Can you work these out from the model? Positions are in its coordinate system, mm. A direction names the side the tool comes from. Give positions to 0.01 mm unless a question says otherwise; leave off trailing zeros. Loops run counter-clockwise (first coordinate to the right, second up) from the corner with the lowest first, then second, coordinate; pieces in that order, holes last. Notation, with made-up numbers: (18.5, -25) - (51.5, -25) arc R34 ccw to (51.5, 14) - close; hole circle Ø11 at (34.25, 75.25). An arc over 180 degrees is marked (long way). Answer in a Markdown table with one row per item.
from build123d import *

# Parameters (mm, degrees)
BOSS_EXTRUDE1_DEPTH = 3.3
BOSS_EXTRUDE2_DEPTH = 2
SKETCH5_W           = 10
SKETCH5_H           = 1.55
BOSS_EXTRUDE3_DEPTH = 0.45
SKETCH6_W           = 10
SKETCH6_H           = 1.55
BOSS_EXTRUDE4_DEPTH = 0.45
SKETCH7_W           = 10
SKETCH7_H           = 1.55
BOSS_EXTRUDE5_DEPTH = 0.45
SKETCH8_W           = 10
SKETCH8_H           = 1.55
BOSS_EXTRUDE6_DEPTH = 0.45
SKETCH9_W           = 30
SKETCH9_H           = 1.55
BOSS_EXTRUDE7_DEPTH = 0.45
SKETCH10_W          = 10
SKETCH10_H          = 1.55
BOSS_EXTRUDE8_DEPTH = 0.45
CHAMFER1_SIZE       = 0.2
SKETCH11_W          = 37.2
SKETCH11_H          = 23
CUT_EXTRUDE1_DEPTH  = 1.6
FILLET1_R           = 0.2


with BuildPart() as part:
    # Sketch1 → Boss-Extrude1 (new body)
    with BuildSketch(Plane(origin=(0, 0, 0), x_dir=(1, 0, 0), z_dir=(0, 1, 0))):
        with BuildLine():
            Line((19.586290833, 59.977163541), (19.586290833, 47.727163541))
            ThreePointArc((19.586290833, 47.727163541), (18.956570412, 46.206883961), (17.436290833, 45.577163541))
            Line((17.436290833, 45.577163541), (-0.413709167, 45.577163541))
            Line((-0.413709167, 45.577163541), (-0.413709167, 5.877163541))
            Line((-0.413709167, 5.877163541), (80.286290833, 5.877163541))
            Line((80.286290833, 5.877163541), (80.286290833, 45.577163541))
            Line((80.286290833, 45.577163541), (62.436290833, 45.577163541))
            ThreePointArc((62.436290833, 45.577163541), (60.916011253, 46.206883961), (60.286290833, 47.727163541))
            Line((60.286290833, 47.727163541), (60.286290833, 59.977163541))
            ThreePointArc((60.286290833, 59.977163541), (59.744438378, 61.285311086), (58.436290833, 61.827163541))
            Line((58.436290833, 61.827163541), (21.436290833, 61.827163541))
            ThreePointArc((21.436290833, 61.827163541), (20.128143288, 61.285311086), (19.586290833, 59.977163541))
        make_face()
    extrude(amount=BOSS_EXTRUDE1_DEPTH)

    # Sketch2 → Boss-Extrude2 (add)
    with BuildSketch(Plane(origin=(0, 3.3, 0), x_dir=(1, 0, 0), z_dir=(0, 1, 0))):
        with BuildLine():
            Line((57.136290833, -1.272836459), (65.436290833, -1.272836459))
            Line((65.436290833, -1.272836459), (80.761323353, 1.251286544))
            ThreePointArc((80.761323353, 1.251286544), (81.961096565, 1.930492929), (82.436290833, 3.224698275))
            Line((82.436290833, 3.224698275), (82.436290833, 45.727163541))
            ThreePointArc((82.436290833, 45.727163541), (81.850504395, 47.141377103), (80.436290833, 47.727163541))
            Line((80.436290833, 47.727163541), (66.436290833, 47.727163541))
            Line((66.436290833, 47.727163541), (62.436290833, 47.727163541))
            Line((62.436290833, 47.727163541), (62.436290833, 61.977163541))
            ThreePointArc((62.436290833, 61.977163541), (61.850504395, 63.391377103), (60.436290833, 63.977163541))
            Line((60.436290833, 63.977163541), (19.436290833, 63.977163541))
            ThreePointArc((19.436290833, 63.977163541), (18.022077271, 63.391377103), (17.436290833, 61.977163541))
            Line((17.436290833, 61.977163541), (17.436290833, 47.727163541))
            Line((17.436290833, 47.727163541), (3.436290833, 47.727163541))
            Line((3.436290833, 47.727163541), (-0.563709167, 47.727163541))
            ThreePointArc((-0.563709167, 47.727163541), (-1.977922729, 47.141377103), (-2.563709167, 45.727163541))
            Line((-2.563709167, 45.727163541), (-2.563709167, -0.472836459))
            ThreePointArc((-2.563709167, -0.472836459), (-2.329394592, -1.038521884), (-1.763709167, -1.272836459))
            Line((-1.763709167, -1.272836459), (21.636290833, -1.272836459))
            ThreePointArc((21.636290833, -1.272836459), (22.201976258, -1.038521884), (22.436290833, -0.472836459))
            Line((22.436290833, -0.472836459), (22.436290833, 3.727163541))
            Line((22.436290833, 3.727163541), (59.036290833, 3.727163541))
            Line((59.036290833, 3.727163541), (59.036290833, 2.703556743))
            Line((59.036290833, 2.703556743), (56.536290833, 1.453556743))
            Line((56.536290833, 1.453556743), (56.536290833, -1.001986721))
            ThreePointArc((56.536290833, -1.001986721), (56.807140571, -1.201986721), (57.136290833, -1.272836459))
        make_face()
    extrude(amount=BOSS_EXTRUDE2_DEPTH)

    # Sketch5 → Boss-Extrude3 (add)
    with BuildSketch(Plane(origin=(0, 0, -45.577163541), x_dir=(-1, 0, 0), z_dir=(0, 0, -1))):
        with Locations((-71.436290833, 1.025)):
            Rectangle(SKETCH5_W, SKETCH5_H)
        with Locations((-8.436290833, 1.025)):
            Rectangle(SKETCH5_W, SKETCH5_H)
    extrude(amount=BOSS_EXTRUDE3_DEPTH)

    # Sketch6 → Boss-Extrude4 (add)
    with BuildSketch(Plane(origin=(0, 0, -61.827163541), x_dir=(-1, 0, 0), z_dir=(0, 0, -1))):
        with Locations((-39.936290833, 1.025)):
            Rectangle(SKETCH6_W, SKETCH6_H)
    extrude(amount=BOSS_EXTRUDE4_DEPTH)

    # Sketch7 → Boss-Extrude5 (add)
    with BuildSketch(Plane(origin=(-0.413709167, 0, 0.363709167), x_dir=(0, 0, 1), z_dir=(-1, 0, 0))):
        with Locations((-26.090872708, 1.025)):
            Rectangle(SKETCH7_W, SKETCH7_H)
    extrude(amount=BOSS_EXTRUDE5_DEPTH)

    # Sketch8 → Boss-Extrude6 (add)
    with BuildSketch(Plane(origin=(80.286290833, 0, -80.236290833), x_dir=(0, 0, 1), z_dir=(-1, 0, 0))):
        with Locations((54.509127292, 1.025)):
            Rectangle(SKETCH8_W, SKETCH8_H)
    extrude(amount=BOSS_EXTRUDE6_DEPTH)

    # Sketch9 → Boss-Extrude7 (add)
    with BuildSketch(Plane.XY.offset(-5.877163541)):
        with Locations((39.936290833, 1.025)):
            Rectangle(SKETCH9_W, SKETCH9_H)
    extrude(amount=BOSS_EXTRUDE7_DEPTH)

    # Sketch10 → Boss-Extrude8 (add)
    with BuildSketch(Plane(origin=(80.286290833, 0, 0), x_dir=(0, 0, -1), z_dir=(1, 0, 0))):
        with Locations((25.727163541, 1.025)):
            Rectangle(SKETCH10_W, SKETCH10_H)
    extrude(amount=BOSS_EXTRUDE8_DEPTH)

    # Chamfer1
    chamfer1_edges = [part.edges().sort_by_distance(p)[0] for p in [
        (8.436290833, 1.8, -46.027163541),
        (8.436290833, 0.25, -46.027163541),
        (39.936290833, 0.25, -62.277163541),
        (39.936290833, 1.8, -62.277163541),
        (-0.863709167, 0.25, -25.727163541),
        (-0.863709167, 1.8, -25.727163541),
        (39.936290833, 1.8, -5.427163541),
        (39.936290833, 0.25, -5.427163541),
        (80.736290833, 0.25, -25.727163541),
        (80.736290833, 1.8, -25.727163541),
        (71.436290833, 0.25, -46.027163541),
        (71.436290833, 1.8, -46.027163541),
    ]]
    chamfer(chamfer1_edges, length=CHAMFER1_SIZE)

    # Sketch11 → Cut-Extrude1 (cut)
    with BuildSketch(Plane(origin=(0, 0, 0), x_dir=(-1, 0, 0), z_dir=(0, -1, 0))):
        with Locations((-29.296290833, 28.397163541)):
            Rectangle(SKETCH11_W, SKETCH11_H)
    extrude(amount=-CUT_EXTRUDE1_DEPTH, mode=Mode.SUBTRACT)

    # Fillet1
    fillet1_edges = [part.edges().sort_by_distance(p)[0] for p in [
        (19.586290833, 0, -53.852163541),
        (20.128143288, 0, -61.285311086),
        (39.936290833, 0, -61.827163541),
        (59.744438378, 0, -61.285311086),
        (60.286290833, 0, -53.852163541),
        (60.916011253, 0, -46.206883961),
        (71.361290833, 0, -45.577163541),
        (80.286290833, 0, -25.727163541),
        (39.936290833, 0, -5.877163541),
        (-0.413709167, 0, -25.727163541),
        (8.511290833, 0, -45.577163541),
        (18.956570412, 0, -46.206883961),
        (29.296290833, 0, -16.897163541),
        (10.696290833, 0, -28.397163541),
        (29.296290833, 0, -39.897163541),
        (47.896290833, 0, -28.397163541),
    ]]
    fillet(fillet1_edges, radius=FILLET1_R)


solid = part.part
Q1. Imagine slicing it at A-A, the plane z = -12.5. Write out the boundary of the cut face in (x, y), and give its area (3 significant figures).
Checked values:
| item | result |
|---|---|
| outline | (-2.56, 3.3) - (-0.41, 3.3) - (-0.41, 0.2) arc R0.2 ccw to (-0.21, 0) - (80.09, 0) arc R0.2 ccw to (80.29, 0.2) - (80.29, 3.3) - (82.44, 3.3) - (82.44, 5.3) - (-2.56, 5.3) - close |
| area | 436 mm² |
Q2. If we mould it in two halves opening along X, with no side actions, what happens to faces 6 (the face through (40, 2, -61.827)), 7 (the face through (-1.96, 4.29, -47.16)), 8 (the face through (56.536, 4, 0))? For each: released by +X, released by -X, zero draft, split by the parting line, or undercut.
Checked values:
| item | result |
|---|---|
| face 6 | zero draft |
| face 7 | released by -X |
| face 8 | undercut |
Q3. Imagine slicing it at D-D, the plane x = 77.5. Write out the boundary of the cut face in (y, z), and give its area (3 significant figures).
Checked values:
| item | result |
|---|---|
| outline | (0, -45.38) arc R0.2 ccw to (0.2, -45.58) - (3.3, -45.58) - (3.3, -47.73) - (5.3, -47.73) - (5.3, -0.71) - (3.3, -0.71) - (3.3, -5.88) - (0.2, -5.88) arc R0.2 ccw to (0, -6.08) - close |
| area | 225 mm² |
Q4. Imagine slicing it at B-B, the plane x = 24. Write out the boundary of the cut face in (y, z).
Checked values:
| item | result |
|---|---|
| outline | (0, -61.63) arc R0.2 ccw to (0.2, -61.83) - (3.3, -61.83) - (3.3, -63.98) - (5.3, -63.98) - (5.3, -3.73) - (3.3, -3.73) - (3.3, -5.88) - (0.2, -5.88) arc R0.2 ccw to (0, -6.08) - (0, -16.7) arc R0.2 ccw to (0.2, -16.9) - (1.6, -16.9) - (1.6, -39.9) - (0.2, -39.9) arc R0.2 ccw to (0, -40.1) - close |
Q5. Imagine slicing it at C-C, the plane x = 9.5. Write out the boundary of the cut face in (y, z), and give its area (3 significant figures).
Checked values:
| item | result |
|---|---|
| outline | (0, -45.38) arc R0.2 ccw to (0.2, -45.58) - (0.25, -45.58) - (0.25, -45.83) - (0.45, -46.03) - (1.6, -46.03) - (1.8, -45.83) - (1.8, -45.58) - (3.3, -45.58) - (3.3, -47.73) - (5.3, -47.73) - (5.3, 1.27) - (3.3, 1.27) - (3.3, -5.88) - (0.2, -5.88) arc R0.2 ccw to (0, -6.08) - close |
| area | 230 mm² |
Q6. On a 3-axis mill with a long thin cutter (end or side, diameter ignored), from which of +Z, -Z, +X, -X, +Y, -Y can I reach the whole of each face in a straight line? I mean faces 1 (the face through (72, 4, -47.727)), 2 (the face through (60.286, 2, -54)), 3 (the face through (18.97, 1.73, -46.22)), 4 (the face through (81.95, 4.29, -1.92)), 5 (the face through (40, 4, -63.977)). Say none if no direction works.
Checked values:
| item | result |
|---|---|
| face 1 | -Z, +X, +Y, -Y |
| face 2 | -Z, +X, -Y |
| face 3 | -Z, -Y |
| face 4 | +Z, +X, +Y, -Y |
| face 5 | -Z, +X, -X, +Y, -Y |
Q7. For pin 1 (2 mm diameter, centred on x = 65, y = 2, fed in from -Z); pin 2 (0.7 mm diameter, centred on x = 36, y = 0.5, fed in from +Z); pin 3 (0.9 mm diameter, centred on y = 2, z = -55, fed in from -X), each with a flat end and sliding along its axis, tell me the tip position at first contact or that it passes through.
Checked values:
| item | result |
|---|---|
| pin 1 | stops at z = -45.58 |
| pin 2 | stops at z = -5.43 |
| pin 3 | stops at x = 19.59 |
Q8. If I drill on line 1 (Z direction, x = 22, y = 1); line 2 (Z direction, x = 28.5, y = 3.25); line 3 (X direction, y = 2.45, z = -49), over which ranges is the centre line in solid material (lowest first)? Write a range as [from, to].
Checked values:
| item | result |
|---|---|
| line 1 | z = [-61.83, -39.9], [-16.9, -5.88] |
| line 2 | z = [-61.83, -5.88] |
| line 3 | x = [19.59, 60.29] |
